from build123d import *

# Parameters (mm, degrees)
SKETCH1_R           = 1.778
SKETCH1_R_2         = 2.794
BASE_DEPTH          = 3.81
SKETCH2_R           = 5.08
SKETCH2_R_2         = 3.2385
BOSS_EXTRUDE2_DEPTH = 3.81


with BuildPart() as part:
    # Sketch1 → base (new body)
    with BuildSketch(Plane(origin=(0, 0, 0), x_dir=(1, 0, 0), z_dir=(0, 1, 0))):
        with BuildLine():
            Line((-5.08, 0), (-5.08, 12.7))
            ThreePointArc((-5.08, 12.7), (0, 17.78), (5.08, 12.7))
            Line((5.08, 12.7), (5.08, 0))
            ThreePointArc((5.08, 0), (0, -5.08), (-5.08, 0))
        make_face()
        with Locations(Location((0, 0, 0), (0, 0, 90))):
            Circle(SKETCH1_R, mode=Mode.SUBTRACT)
        with Locations(Location((0, 12.7, 0), (0, 0, 90))):
            Circle(SKETCH1_R_2, mode=Mode.SUBTRACT)
    extrude(amount=BASE_DEPTH)

    # Sketch2 → Boss-Extrude2 (add)
    with BuildSketch(Plane(origin=(0, 3.81, 0), x_dir=(1, 0, 0), z_dir=(0, 1, 0))):
        Circle(SKETCH2_R)
        with Locations(Location((0, 0, 0), (0, 0, 90))):
            Circle(SKETCH2_R_2, mode=Mode.SUBTRACT)
    extrude(amount=BOSS_EXTRUDE2_DEPTH)


solid = part.part
Design review of the part built by this model. Coordinates are the model's own, in mm. A direction names the side the tool comes from. Coordinates: 2 decimals unless noted, no trailing zeros. Loops run counter-clockwise (first coordinate to the right, second up) from the corner with the lowest first, then second, coordinate; pieces in that order, holes last.
Item 1: Wall thickness on L1, parallel to X at y = 2.5, z = 0; L2, parallel to Z at x = 1, y = 0.75; L3, parallel to X at y = 1.25, z = -12.7: over which ranges is each line inside the solid? List them lowest first.
Completed:
L1: x = -5.08 to -1.78, 1.78 to 5.08
L2: z = -17.68 to -15.31, -10.09 to -1.47, 1.47 to 4.98
L3: x = -5.08 to -2.79, 2.79 to 5.08
Item 2: For faces 1 (the flat face through (-1.4, 3.81, 1.4)), 2 (the flat face through (0, 0, -7)), list the 3-axis set-ups (+Z, -Z, +X, -X, +Y, -Y) from which the entire face can be reached by the end or side of a thin tool; tool diameter is ignored.
Completed:
face 1: +Y
face 2: +Z, -Z, +X, -X, -Y
Item 3: Draft analysis for pull direction X (two halves, no side actions). For faces 3 (the flat face through (0, 3.81, -9)), 4 (the cylindrical face through (3.16, 5.69, 0.7)), 5 (the cylindrical face through (-0.11, 1.88, -17.78)), state which applies: pulls with the +X half, pulls with the -X half, needs draft (parallel to the pull), parting line crosses it, or undercut.
Completed:
face 3: needs draft
face 4: undercut
face 5: parting line crosses it
Item 4: Add section C-C (y = 4.5). Write out the cut boundary in (x, z), and give its area (3 significant figures).
Completed:
outline: circle Ø10.16 at (0, 0); hole circle Ø6.48 at (0, 0)
area: 48.1 mm2
Item 5: Add section B-B (z = -11). Write out the cut boundary in (x, y).
Completed:
outline: (-5.08, 0) - (-2.22, 0) - (-2.22, 3.81) - (-5.08, 3.81) - close; (2.22, 0) - (5.08, 0) - (5.08, 3.81) - (2.22, 3.81) - close
Item 6: Clearance check with flat-ended pins moving along their axes: pin 1 (4 mm diameter, centred on x = 0, z = 0, fed in from +Y); pin 2 (1 mm diameter, centred on x = -1.5, z = -11.5, fed in from -Y). State where each tip first meets the part, or that it passes through.
Completed:
pin 1: stops at y = 3.81
pin 2: passes through
Item 7: Add section A-A (x = 0). Write out the cut boundary in (y, z), and give its area (3 significant figures).
Completed:
outline: (0, -17.78) - (3.81, -17.78) - (3.81, -15.49) - (0, -15.49) - close; (0, -9.91) - (3.81, -9.91) - (3.81, -5.08) - (7.62, -5.08) - (7.62, -3.24) - (3.81, -3.24) - (3.81, -1.78) - (0, -1.78) - close; (0, 1.78) - (3.81, 1.78) - (3.81, 3.24) - (7.62, 3.24) - (7.62, 5.08) - (0, 5.08) - close
area: 66.3 mm2
Item 8: Add section D-D (z = -6.75). Write out the cut boundary in (x, y), and give its area (3 significant figures).
Completed:
outline: (-5.08, 0) - (5.08, 0) - (5.08, 3.81) - (-5.08, 3.81) - close
area: 38.7 mm2
